from build123d import *

# Parameters (mm, degrees)
F1_DEPTH  = 20
F2_R      = 8.175018
F2_R_2    = 3.780512
F3_DEPTH  = 1
F3_FACE_R = 3.780512
F4_DEPTH  = 47.6
F5_R      = 5


with BuildPart() as f1:
    # F0 (on Front) → F1 (new body)
    with BuildSketch(Plane.XZ):
        with BuildLine():
            ThreePointArc((12, 5), (0, -13), (-12, 5))
            Line((-12, 5), (-12, 31))
            Line((-12, 31), (-15, 31))
            Line((-15, 31), (-15, 0))
            ThreePointArc((-15, 0), (0, -15), (15, 0))
            Line((15, 0), (15, 31))
            Line((15, 31), (12, 31))
            Line((12, 31), (12, 5))
        make_face()
    extrude(amount=F1_DEPTH)

    # F2 (on face) → F3 (join)
    with BuildSketch(Plane(origin=(-15, 0, 0), x_dir=(0, -1, 0), z_dir=(-1, 0, 0))):
        with Locations((10, 15.762184)):
            Circle(F2_R)
        with Locations((10, 15.762184)):
            Circle(F2_R_2, mode=Mode.SUBTRACT)
    extrude(amount=F3_DEPTH)

    # F3_face (on face) → F4 (cut)
    with BuildSketch(Plane(origin=(-15, -10, 15.762184), x_dir=(0, -1, 0), z_dir=(-1, 0, 0))):
        Circle(F3_FACE_R)
    extrude(amount=-F4_DEPTH, mode=Mode.SUBTRACT)

    # F5
    f5_edges = [f1.edges().sort_by_distance(p)[0] for p in [
        (-13.5, -20, 31),
        (-13.5, 0, 31),
        (13.5, -20, 31),
        (13.5, 0, 31),
    ]]
    fillet(f5_edges, radius=F5_R)


solid = f1.part
Can you work these out from the model? Positions are in its coordinate system, mm. A direction names the side the tool comes from. Coordinates: 2 decimals unless noted, no trailing zeros. Order: outer loops, then holes, each group sorted by start corner. A loop starts at its lowest first (then second) coordinate and runs counter-clockwise, first axis right, second up. Notation, with made-up numbers: (55, -22) - (109, -22) arc R30 ccw to (109, 13) - close; hole circle Ø5 at (88.25, 38). An arc over 180 degrees is marked (long way). Answer as a JSON object with one key per item and string values. Group by question number.
Q1. Imagine slicing it at B-B (z = -5). Please give me the cut outline in (x, y), and give its area (3 significant figures).
Q2. Will these pins go through, and if not, where does the flat tip stop? P1, Ø3, axis at x = -12.5, z = 3.5, coming from the +Y side; P2, Ø5, axis at y = -15.5, z = -4.5, coming from the +X side.
Q3. Imagine slicing it at D-D (y = -4). Please give me the cut outline in (x, z).
Q4. Imagine slicing it at C-C (z = 15). Please give me the cut outline in (x, y), and give its area (3 significant figures).
Q5. We'd pull the mould along X, two halves only. Please class faces 1 (the face through (-12, -10, 21)), 2 (the face through (-16, -12, 12)), 3 (the face through (12, -10, 21)), 4 (the face through (-15.49, -8.23, 7.78)): +X half, -X half, draft (parallel to the pull), parting line (faces both ways), or undercut.
Q6. On a 3-axis mill with a long thin cutter (end or side, diameter ignored), from which of +Z, -Z, +X, -X, +Y, -Y can I reach the whole of each face in a straight line? I mean faces 5 (the face through (14, -10, 31)), 6 (the face through (-15, -5, 9)). Say none if no direction works.
Q7. I need wall thicknesses on line 1 (X direction, y = -5.5, z = -0.5); line 2 (X direction, y = -11, z = 8); line 3 (Z direction, x = -15.25, y = -10). Which ranges of each line are inside material? Lowest first, please. Write a range as from..to.
Q8. Imagine slicing it at A-A (y = -10). Please give me the cut outline in (x, z), and give its area (3 significant figures).
Determined:
{
 "1": {"outline": "(-14.14, -20) - (-12, -20) - (-12, 0) - (-14.14, 0) - close; (12, -20) - (14.14, -20) - (14.14, 0) - (12, 0) - close", "area": "85.7 mm2"},
 "2": {"P1": "stops at y = 0", "P2": "stops at x = 14.87"},
 "3": {"outline": "(-16, 10.21) - (-15, 10.21) - (-15, 0) arc R15 ccw to (15, 0) - (15, 30.9) - (12, 30.9) - (12, 5) arc R13 cw (long way) to (-12, 5) - (-12, 30.9) - (-15, 30.9) - (-15, 21.31) - (-16, 21.31) - close"},
 "4": {"outline": "(-16, -18.14) - (-15, -18.14) - (-15, -20) - (-12, -20) - (-12, -13.7) - (-16, -13.7) - close; (-16, -6.3) - (-12, -6.3) - (-12, 0) - (-15, 0) - (-15, -1.86) - (-16, -1.86) - close; (12, -20) - (15, -20) - (15, -13.7) - (12, -13.7) - close; (12, -6.3) - (15, -6.3) - (15, 0) - (12, 0) - close", "area": "84.4 mm2"},
 "5": {"face 1": "undercut", "face 2": "-X half", "face 3": "undercut", "face 4": "draft"},
 "6": {"face 5": "+Z, +X, -X, +Y, -Y", "face 6": "-X"},
 "7": {"line 1": "x = -14.99..-12.99, 12.99..14.99", "line 2": "x = -16..-12, 12..15", "line 3": "z = 7.59..11.98, 19.54..23.94"},
 "8": {"outline": "(-16, 7.59) - (-15, 7.59) - (-15, 0) arc R15 ccw to (15, 0) - (15, 11.98) - (12, 11.98) - (12, 5) arc R13 cw (long way) to (-12, 5) - (-12, 11.98) - (-16, 11.98) - close; (-16, 19.54) - (-12, 19.54) - (-12, 31) - (-15, 31) - (-15, 23.94) - (-16, 23.94) - close; (12, 19.54) - (15, 19.54) - (15, 31) - (12, 31) - close", "area": "231 mm2"}
}
